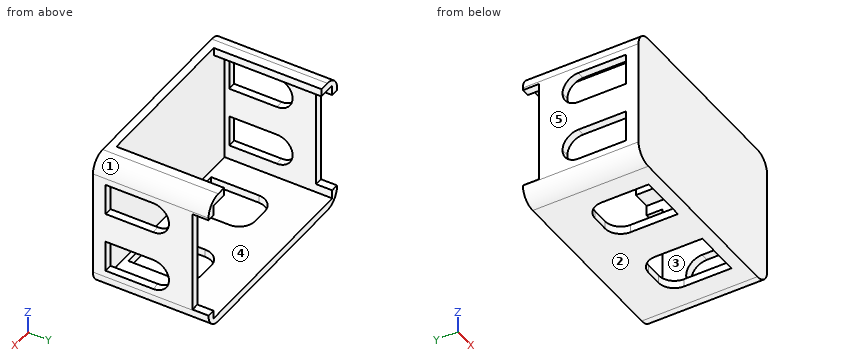
```python
from build123d import *

# Parameters (mm, degrees)
SKETCH1_W               = 132
SKETCH1_H               = 87.5
BOSS_EXTRUDE1_DEPTH     = 5
BOSS_EXTRUDE2_DEPTH     = 68
CUT_EXTRUDE1_DEPTH      = 175.382481918
CUT_EXTRUDE1_DEPTH_BACK = 175.382481918
SKETCH3_W               = 20
SKETCH3_H               = 40
CUT_EXTRUDE2_REACH      = 176.382
SKETCH4_W               = 30
SKETCH4_H               = 40
SKETCH5_W               = 65.5
SKETCH5_H               = 10.1
CUT_EXTRUDE3_DEPTH      = 175.382481918
FILLET1_R               = 10


with BuildPart() as part:
    # Sketch1 → Boss-Extrude1 (new body)
    with BuildSketch(Plane(origin=(0, 0, 0), x_dir=(1, 0, 0), z_dir=(0, 1, 0))):
        with Locations((66, 43.75)):
            Rectangle(SKETCH1_W, SKETCH1_H)
    extrude(amount=BOSS_EXTRUDE1_DEPTH)

    # Sketch2 → Boss-Extrude2 (add)
    with BuildSketch(Plane(origin=(0, 5, 0), x_dir=(1, 0, 0), z_dir=(0, 1, 0))):
        Polygon((5, 5), (16, 5), (16, 0), (0, 0), (0, 87.5), (132, 87.5), (132, 0), (116, 0), (116, 5), (127, 5), (127, 82.5), (5, 82.5), align=None)
    extrude(amount=BOSS_EXTRUDE2_DEPTH)

    # Sketch3 → Cut-Extrude1 (cut, two sides: drawn at the far end of the back side and taken through both)
    with BuildSketch(Plane(origin=(132, 0, 0), x_dir=(0, 0, -1), z_dir=(1, 0, 0)).offset(-CUT_EXTRUDE1_DEPTH_BACK)):
        with Locations((24.25, 28)):
            Rectangle(SKETCH3_W, SKETCH3_H)
        with Locations((63.25, 28)):
            Rectangle(SKETCH3_W, SKETCH3_H)
    extrude(amount=CUT_EXTRUDE1_DEPTH + CUT_EXTRUDE1_DEPTH_BACK, mode=Mode.SUBTRACT)

    # Sketch4 → Cut-Extrude2 (cut, up to next)
    with BuildSketch(Plane(origin=(0, 0, -87.5), x_dir=(-1, 0, 0), z_dir=(0, 0, -1)), mode=Mode.PRIVATE) as cut_extrude2_sk1:
        with Locations((-93.5, 28)):
            Rectangle(SKETCH4_W, SKETCH4_H)
    cut_extrude2_tool1 = extrude(cut_extrude2_sk1.sketch, amount=-CUT_EXTRUDE2_REACH, mode=Mode.PRIVATE) & part.part
    # Sketch4 → Cut-Extrude2 (cut, up to next)
    with BuildSketch(Plane(origin=(0, 0, -87.5), x_dir=(-1, 0, 0), z_dir=(0, 0, -1)), mode=Mode.PRIVATE) as cut_extrude2_sk2:
        with Locations((-38.5, 28)):
            Rectangle(SKETCH4_W, SKETCH4_H)
    cut_extrude2_tool2 = extrude(cut_extrude2_sk2.sketch, amount=-CUT_EXTRUDE2_REACH, mode=Mode.PRIVATE) & part.part
    add(cut_extrude2_tool1.solids().sort_by_distance((93.5, 28, -87.5))[0], mode=Mode.SUBTRACT)
    add(cut_extrude2_tool2.solids().sort_by_distance((38.5, 28, -87.5))[0], mode=Mode.SUBTRACT)

    # Sketch5 → Cut-Extrude3 (cut, through all)
    with BuildSketch(Plane.ZY):
        with Locations((-44.2623336, 67.95)):
            Rectangle(SKETCH5_W, SKETCH5_H)
    extrude(amount=-CUT_EXTRUDE3_DEPTH, mode=Mode.SUBTRACT)

    # Fillet1
    fillet1_edges = [part.edges().sort_by_distance(p)[0] for p in [
        (108.5, 48, -85),
        (78.5, 48, -85),
        (53.5, 48, -85),
        (23.5, 48, -85),
        (2.5, 48, -73.25),
        (2.5, 48, -53.25),
        (2.5, 48, -14.25),
        (2.5, 48, -34.25),
        (129.5, 48, -14.25),
        (129.5, 48, -34.25),
        (129.5, 48, -73.25),
        (129.5, 48, -53.25),
        (132, 36.5, -87.5),
        (132, 36.5, 0),
        (0, 36.5, 0),
        (0, 36.5, -87.5),
    ]]
    fillet(fillet1_edges, radius=FILLET1_R - 0.0001)  # a hair under: the kernel refuses the full size


solid = part.part
```
Work out the finished part from the listing and answer in its coordinate system (mm). Face numbers are marked on the shaded views. A direction names the side the tool comes from. Coordinates: 2 decimals unless noted, no trailing zeros. Write each loop counter-clockwise with the first axis right and the second up, starting at its lowest first coordinate (ties: lowest second). Pieces come first, ordered by that corner, then holes.
Q1. Find the intervals of material crossed by line 1 (X direction, y = 33, z = -9.5); line 2 (Z direction, x = 61, y = 59); line 3 (Y direction, x = 71.5, z = -21.5), in increasing order.
Q2. A cutting plane is placed at A-A, the plane y = 67. Give the vertices of the cut face in (x, z).
Q3. A cutting plane is placed at D-D, the plane x = 119. Give the vertices of the cut face in (y, z).
Q4. Which of the six approach directions +Z, -Z, +X, -X, +Y, -Y give full straight-line access (tool end or side, diameter ignored) to the marked faces 4 and 5?
Q5. A cutting plane is placed at B-B, the plane z = -21. Give the vertices of the cut face in (x, y).
Q6. Each of these flat-tipped pins is pushed along its axis until it touches: pin 1 Ø4 at (x, z) = (130, -21.5) entering from +Y; pin 2 Ø12 at (x, y) = (57.5, 44.5) entering from +Z; pin 3 Ø4 at (x, y) = (130.5, 66.5) entering from -Z. Where does it stop, or does it pass through?
Q7. Determine the mould class of the marked faces 1, 2 and 3 for opening direction X: released by +X, released by -X, zero draft, split by the parting line, or undercut.
Q8. A cutting plane is placed at C-C, the plane y = 52.5. Give the vertices of the cut face in (x, z), then the cut area to 3 significant figures.
Findings below:
1. line 1: x = 0.01 to 5, 127 to 131.99
1. line 2: z = -87.5 to -82.5
1. line 3: y = 0 to 5
2. outline: (0, -77.5) arc R10 ccw to (10, -87.5) - (122, -87.5) arc R10 ccw to (132, -77.5) - (132, -77.01) - (127, -77.01) - (127, -82.5) - (5, -82.5) - (5, -77.01) - (0, -77.01) - close; (0, -11.51) - (5, -11.51) - (5, -5) - (16, -5) - (16, 0) - (10, 0) arc R10 ccw to (0, -10) - close; (116, -5) - (127, -5) - (127, -11.51) - (132, -11.51) - (132, -10) arc R10 ccw to (122, 0) - (116, 0) - close
3. outline: (0, -87.5) - (73, -87.5) - (73, -82.5) - (5, -82.5) - (5, -5) - (73, -5) - (73, 0) - (0, 0) - close
4. face 4: +Y
4. face 5: +Z, -Z, -X, +Y, -Y
5. outline: (0, 0) - (132, 0) - (132, 8) - (127, 8) - (127, 5) - (5, 5) - (5, 8) - (0, 8) - close; (0, 47.46) - (5, 47.46) - (5, 62.9) - (0, 62.9) - close; (127, 47.46) - (132, 47.46) - (132, 62.9) - (127, 62.9) - close
6. pin 1: stops at y = 62.9
6. pin 2: stops at z = -82.5
6. pin 3: stops at z = -85.1
7. face 1: released by +X
7. face 2: zero draft
7. face 3: undercut
8. outline: (0, -77.5) arc R10 ccw to (10, -87.5) - (122, -87.5) arc R10 ccw to (132, -77.5) - (132, -10) arc R10 ccw to (122, 0) - (116, 0) - (116, -5) - (127, -5) - (127, -82.5) - (5, -82.5) - (5, -5) - (16, -5) - (16, 0) - (10, 0) arc R10 ccw to (0, -10) - close
8. area: 1,510 mm2
